from build123d import *

# Parameters (mm, degrees)
SKETCH1_W           = 25.4
SKETCH1_H           = 50.8
SKETCH1_W_2         = 22.225
SKETCH1_H_2         = 47.625
BOSS_EXTRUDE1_DEPTH = 660.4
SKETCH2_R           = 2.54
SKETCH2_R_2         = 14.2875
CUT_EXTRUDE1_DEPTH  = 662.376201568
SKETCH3_R           = 2.54
CUT_EXTRUDE3_DEPTH  = 663.472708872


with BuildPart() as part:
    # Sketch1 → Boss-Extrude1 (new body)
    with BuildSketch(Plane.XY):
        Rectangle(SKETCH1_W, SKETCH1_H)
        Rectangle(SKETCH1_W_2, SKETCH1_H_2, mode=Mode.SUBTRACT)
    extrude(amount=BOSS_EXTRUDE1_DEPTH)

    # Sketch2 → Cut-Extrude1 (cut, through all)
    with BuildSketch(Plane(origin=(12.7, 0, 0), x_dir=(0, 0, -1), z_dir=(1, 0, 0))):
        with Locations((-38.1, 9.525)):
            Circle(SKETCH2_R)
        with Locations((-38.1, -12.7)):
            Circle(SKETCH2_R)
        with Locations((-12.7, 9.525)):
            Circle(SKETCH2_R)
        with Locations((-12.7, -12.7)):
            Circle(SKETCH2_R)
        with Locations((-152.4, 0)):
            Circle(SKETCH2_R_2)
        with Locations((-644.525, -12.7)):
            Circle(SKETCH2_R)
        with Locations((-622.3, -12.7)):
            Circle(SKETCH2_R)
        with Locations((-644.525, 12.7)):
            Circle(SKETCH2_R)
        with Locations((-622.3, 12.7)):
            Circle(SKETCH2_R)
        with Locations((-25.4, 0)):
            Circle(SKETCH2_R)
        with Locations((-76.2, 0)):
            Circle(SKETCH2_R)
        with Locations((-127, 0)):
            Circle(SKETCH2_R)
        with Locations((-177.8, 0)):
            Circle(SKETCH2_R)
        with Locations((-228.6, 0)):
            Circle(SKETCH2_R)
        with Locations((-279.4, 0)):
            Circle(SKETCH2_R)
        with Locations((-330.2, 0)):
            Circle(SKETCH2_R)
        with Locations((-381, 0)):
            Circle(SKETCH2_R)
        with Locations((-431.8, 0)):
            Circle(SKETCH2_R)
        with Locations((-482.6, 0)):
            Circle(SKETCH2_R)
        with Locations((-533.4, 0)):
            Circle(SKETCH2_R)
        with Locations((-584.2, 0)):
            Circle(SKETCH2_R)
    extrude(amount=-CUT_EXTRUDE1_DEPTH, mode=Mode.SUBTRACT)

    # Sketch3 → Cut-Extrude3 (cut, through all)
    with BuildSketch(Plane(origin=(0, 25.4, 0), x_dir=(1, 0, 0), z_dir=(0, 1, 0))):
        with Locations(Location((0, -12.7, 0), (0, 0, 270))):
            Circle(SKETCH3_R)
        with Locations(Location((0, -38.1, 0), (0, 0, 270))):
            Circle(SKETCH3_R)
        with Locations(Location((0, -622.3, 0), (0, 0, 270))):
            Circle(SKETCH3_R)
        with Locations(Location((0, -571.5, 0), (0, 0, 270))):
            Circle(SKETCH3_R)
        with Locations(Location((0, -520.7, 0), (0, 0, 270))):
            Circle(SKETCH3_R)
        with Locations(Location((0, -469.9, 0), (0, 0, 270))):
            Circle(SKETCH3_R)
        with Locations(Location((0, -419.1, 0), (0, 0, 270))):
            Circle(SKETCH3_R)
        with Locations(Location((0, -368.3, 0), (0, 0, 270))):
            Circle(SKETCH3_R)
        with Locations(Location((0, -317.5, 0), (0, 0, 270))):
            Circle(SKETCH3_R)
        with Locations(Location((0, -266.7, 0), (0, 0, 270))):
            Circle(SKETCH3_R)
    extrude(amount=-CUT_EXTRUDE3_DEPTH, mode=Mode.SUBTRACT)


solid = part.part
Design review of the part built by this model. Coordinates are the model's own, in mm. A direction names the side the tool comes from. Round coordinates to 2 decimals unless told otherwise and drop trailing zeros. Order: outer loops, then holes, each group sorted by start corner. A loop starts at its lowest first (then second) coordinate and runs counter-clockwise, first axis right, second up. Notation, with made-up numbers: M -20.75,-24 L -16.75,-24 A26 ccw -16.75,15 Z; hole C 57,-3.75 d5. An arc over 180 degrees is marked long. Answer as CSV lines item,"result". Start each with the question number.
1) Add section A-A (z = 602). Give the boundary of the cut face in (x, y), then the cut area to 3 significant figures.
2) For pin 1 Ø8 at (y, z) = (0, 127) entering from +X, flat-tipped, find the tip position at first contact; note if it passes through.
3) Wall thickness on line 1 along X through (y, z) = (19.5, 291); line 2 along Y through (x, z) = (4, 126); line 3 along X through (y, z) = (-24.55, 520.7): over which ranges is each line inside the solid? List them lowest first. Write a range as [from, to].
4) Tool access review of faces 4 (the face through (-12.7, 0, 326)), 5 (the face through (0, 23.812, 326)): name each direction out of +Z, -Z, +X, -X, +Y, -Y from which nothing blocks a thin tool from reaching the whole face with its end or side.
5) The part is to be moulded in two halves that separate along Z. For faces 1 (the face through (-11.3, 2, 660.4)), 2 (the face through (-11.112, 0, 326)), 3 (the face through (11.92, -5.47, 139.2)), say which applies: +Z half, -Z half, draft (parallel to the pull), parting line (faces both ways), or undercut.
Resolved:
1,outline,"M -12.7,-25.4 L 12.7,-25.4 L 12.7,25.4 L -12.7,25.4 Z; hole M -11.11,-23.81 L 11.11,-23.81 L 11.11,23.81 L -11.11,23.81 Z"
1,area,"232 mm^2"
2,pin 1,"x = 12.7"
3,line 1,"[-12.7, -11.11], [11.11, 12.7]"
3,line 2,"[-25.4, -23.81], [23.81, 25.4]"
3,line 3,"[-12.7, -2.54], [2.54, 12.7]"
4,face 4,"+Z, -Z, -X, +Y, -Y"
4,face 5,"+Z, -Z"
5,face 1,"+Z half"
5,face 2,"draft"
5,face 3,"undercut"
